from build123d import *
from build123d.topology import SkipClean

# Parameters (mm, degrees)
SKETCH1_R                      = 40
SKETCH1_R_2                    = 38
BOSS_EXTRUDE1_DEPTH            = 200
SKETCH2_R                      = 40
BOSS_EXTRUDE2_DEPTH            = 2
BOSS_EXTRUDE3_DEPTH            = 107
BOSS_EXTRUDE4_DEPTH            = 2
SKETCH5_R                      = 1.75
CUT_EXTRUDE1_DEPTH             = 225.428162226
CUT_EXTRUDE2_REACH             = 218.296
SKETCH6_R                      = 4
CUT_EXTRUDE2_DIRECTION_2_REACH = 218.296
CIRPATTERN1_COUNT              = 2
CIRPATTERN1_ANGLE              = 90
BOSS_EXTRUDE5_REACH            = 241.742
BOSS_EXTRUDE5_END_RADIUS       = 40
SKETCH7_W                      = 14
SKETCH7_H                      = 5
CUT_EXTRUDE3_REACH             = 221.818
SKETCH8_R                      = 1.75
FILLET1_R                      = 3
CUT_EXTRUDE4_REACH             = 220.598
SKETCH9_R                      = 0.25
BOSS_EXTRUDE6_START            = 2
BOSS_EXTRUDE6_DEPTH            = 2
CUT_EXTRUDE5_REACH             = 220.147


with BuildPart() as part:
    # Sketch1 → Boss-Extrude1 (new body)
    with BuildSketch(Plane.XY):
        Circle(SKETCH1_R)
        Circle(SKETCH1_R_2, mode=Mode.SUBTRACT)
    extrude(amount=BOSS_EXTRUDE1_DEPTH)

    # Sketch2 → Boss-Extrude2 (add)
    with BuildSketch(Plane.XY.offset(180)):
        Circle(SKETCH2_R)
    extrude(amount=BOSS_EXTRUDE2_DEPTH)

    # Sketch3 → Boss-Extrude3 (add)
    with BuildSketch(Plane(origin=(0, 0, 0), x_dir=(-1, 0, 0), z_dir=(0, 0, -1))):
        with BuildLine():
            Line((-24, -32), (-72, -32))
            Line((-72, -32), (-72, -30))
            Line((-72, -30), (-26.457513111, -30))
            ThreePointArc((-26.457513111, -30), (-25.248567431, -31.024342744), (-24, -32))
        make_face()
        with BuildLine():
            Line((-24, 32), (-72, 32))
            Line((-72, 32), (-72, 30))
            Line((-72, 30), (-26.457513111, 30))
            ThreePointArc((-26.457513111, 30), (-25.248567431, 31.024342744), (-24, 32))
        make_face()
    extrude(amount=-BOSS_EXTRUDE3_DEPTH)

    # Sketch4 → Boss-Extrude4 (add)
    with BuildSketch(Plane.XY.offset(107)):
        with BuildLine():
            Line((72, -32), (24, -32))
            ThreePointArc((24, -32), (40, 0), (24, 32))
            Line((24, 32), (72, 32))
            Line((72, 32), (72, -32))
        make_face()
    extrude(amount=BOSS_EXTRUDE4_DEPTH)

    # Sketch5 → Cut-Extrude1 (cut, through all)
    with BuildSketch(Plane(origin=(0, 32, 0), x_dir=(1, 0, 0), z_dir=(0, 1, 0))):
        with Locations(Location((43.5, -102.5, 0), (0, 0, 270))):
            Circle(SKETCH5_R)
        with Locations(Location((43.5, -3.5, 0), (0, 0, 270))):
            Circle(SKETCH5_R)
        with Locations(Location((68.5, -78, 0), (0, 0, 270))):
            Circle(SKETCH5_R)
    extrude(amount=-CUT_EXTRUDE1_DEPTH, mode=Mode.SUBTRACT)

    # Sketch6 → Cut-Extrude2 (cut, up to next)
    with BuildSketch(Plane(origin=(0, 0, 0), x_dir=(0, 0, 1), z_dir=(-0.7071067811865488, 0.7071067811865464, 0)), mode=Mode.PRIVATE) as cut_extrude2_sk1:
        with Locations(Location((187, 0, 0), (0, 0, 90))):
            Circle(SKETCH6_R)
    cut_extrude2_tool1 = extrude(cut_extrude2_sk1.sketch, amount=-CUT_EXTRUDE2_REACH, mode=Mode.PRIVATE) & part.part
    cut_extrude2 = cut_extrude2_tool1.solids().sort_by_distance((0, 0, 187))[0]
    add(cut_extrude2, mode=Mode.SUBTRACT)

    # Sketch6 → Cut-Extrude2 direction 2 (cut, up to next)
    with BuildSketch(Plane(origin=(0, 0, 0), x_dir=(0, 0, 1), z_dir=(-0.7071067811865488, 0.7071067811865464, 0)), mode=Mode.PRIVATE) as cut_extrude2_direction_2_sk1:
        with Locations(Location((187, 0, 0), (0, 0, 90))):
            Circle(SKETCH6_R)
    cut_extrude2_direction_2_tool1 = extrude(cut_extrude2_direction_2_sk1.sketch, amount=CUT_EXTRUDE2_DIRECTION_2_REACH, mode=Mode.PRIVATE) & part.part
    cut_extrude2_direction_2 = cut_extrude2_direction_2_tool1.solids().sort_by_distance((0, 0, 187))[0]
    add(cut_extrude2_direction_2, mode=Mode.SUBTRACT)

    # CirPattern1: Cut-Extrude2, Cut-Extrude2 direction 2 ×2 about axis
    cirpattern1_axis = Axis((0, 0, -12.1), (0, 0, 1))
    add([cut_extrude2.rotate(cirpattern1_axis, i * CIRPATTERN1_ANGLE / (CIRPATTERN1_COUNT - 1)) for i in range(1, CIRPATTERN1_COUNT)], mode=Mode.SUBTRACT)
    add([cut_extrude2_direction_2.rotate(cirpattern1_axis, i * CIRPATTERN1_ANGLE / (CIRPATTERN1_COUNT - 1)) for i in range(1, CIRPATTERN1_COUNT)], mode=Mode.SUBTRACT)

    # Boss-Extrude5: up to this cylinder (the profile starts outside it)
    boss_extrude5_end = Plane(origin=(0, 0, 7), z_dir=(0, 0, -1)) * Cylinder(BOSS_EXTRUDE5_END_RADIUS, 564.484, mode=Mode.PRIVATE)
    # Sketch7 → Boss-Extrude5 (add, up to the surface)
    with BuildSketch(Plane(origin=(-54, 0, 0), x_dir=(0, 0, -1), z_dir=(1, 0, 0)), mode=Mode.PRIVATE) as boss_extrude5_sk1:
        with Locations((-7, -13.5)):
            Rectangle(SKETCH7_W, SKETCH7_H)
    boss_extrude5_tool1 = extrude(boss_extrude5_sk1.sketch, amount=BOSS_EXTRUDE5_REACH, mode=Mode.PRIVATE) - boss_extrude5_end
    add(boss_extrude5_tool1.solids().sort_by_distance((-54, -13.5, 7))[0])
    # Sketch7 → Boss-Extrude5 (add, up to the surface)
    with BuildSketch(Plane(origin=(-54, 0, 0), x_dir=(0, 0, -1), z_dir=(1, 0, 0)), mode=Mode.PRIVATE) as boss_extrude5_sk2:
        with Locations((-7, 13.5)):
            Rectangle(SKETCH7_W, SKETCH7_H)
    boss_extrude5_tool2 = extrude(boss_extrude5_sk2.sketch, amount=BOSS_EXTRUDE5_REACH, mode=Mode.PRIVATE) - boss_extrude5_end
    add(boss_extrude5_tool2.solids().sort_by_distance((-54, 13.5, 7))[0])

    # Cut-Extrude3: up to this face of the body (flat: up to its plane)
    cut_extrude3_end = Plane(part.part.faces().sort_by_distance((-45.33030278, 16, 7))[0])
    # Sketch8 → Cut-Extrude3 (cut, up to the picked face)
    with BuildSketch(Plane.XZ.offset(16), mode=Mode.PRIVATE) as cut_extrude3_sk1:
        with Locations(Location((-50, 5, 0), (0, 0, 270))):
            Circle(SKETCH8_R)
    cut_extrude3_tool1 = split(extrude(cut_extrude3_sk1.sketch, amount=-CUT_EXTRUDE3_REACH, mode=Mode.PRIVATE), bisect_by=cut_extrude3_end, keep=Keep.BOTH, mode=Mode.PRIVATE)
    add(cut_extrude3_tool1.solids().sort_by(Axis((-50, -16, 5), (0, 1, 0)))[0], mode=Mode.SUBTRACT)

    # Fillet1
    fillet1_edges = [part.edges().sort_by_distance(p)[0] for p in [
        (-54, -13.5, 14),
        (-54, -13.5, 0),
        (-54, 13.5, 0),
        (-54, 13.5, 14),
    ]]
    fillet(fillet1_edges, radius=FILLET1_R)

    # Sketch9 → Cut-Extrude4 (cut, up to next)
    with BuildSketch(Plane.XZ.offset(-11), mode=Mode.PRIVATE) as cut_extrude4_sk1:
        with Locations(Location((-44, 7, 0), (0, 0, 270))):
            Circle(SKETCH9_R)
    cut_extrude4_tool1 = extrude(cut_extrude4_sk1.sketch, amount=-CUT_EXTRUDE4_REACH, mode=Mode.PRIVATE) & part.part
    add(cut_extrude4_tool1.solids().sort_by_distance((-44, 11, 7))[0], mode=Mode.SUBTRACT)

    # Sketch10 → Boss-Extrude6 (add)
    with SkipClean():  # the faces are left unmerged after this step: merging them gives an invalid solid
        with BuildSketch(Plane(origin=(0, 0, 0), x_dir=(-1, 0, 0), z_dir=(0, 0, -1)).offset(BOSS_EXTRUDE6_START)):
            with BuildLine():
                ThreePointArc((10, -36.66060556), (0, -38), (-10, -36.66060556))
                Line((-10, -36.66060556), (-10, -38.729833462))
                ThreePointArc((-10, -38.729833462), (0, -40), (10, -38.729833462))
                Line((10, -38.729833462), (10, -36.66060556))
            make_face()
            with BuildLine():
                ThreePointArc((10, 38.729833462), (0, 40), (-10, 38.729833462))
                Line((-10, 38.729833462), (-10, 36.66060556))
                ThreePointArc((-10, 36.66060556), (0, 38), (10, 36.66060556))
                Line((10, 36.66060556), (10, 38.729833462))
            make_face()
        extrude(amount=-BOSS_EXTRUDE6_DEPTH)

    # Sketch11 → Cut-Extrude5 (cut, up to next)
    with BuildSketch(Plane.XY.offset(200), mode=Mode.PRIVATE) as cut_extrude5_sk1:
        with BuildLine():
            ThreePointArc((14.062684519, 37.446507235), (-20.975291487, 34.059318065), (-39.768785027, 4.294617267))
            ThreePointArc((-39.768785027, 4.294617267), (-57.533773757, -120.199175418), (66.76517374, -101.118533584))
            ThreePointArc((66.76517374, -101.118533584), (210.736936915, 32.945452835), (14.062684519, 37.446507235))
        make_face()
    cut_extrude5_tool1 = extrude(cut_extrude5_sk1.sketch, amount=-CUT_EXTRUDE5_REACH, mode=Mode.PRIVATE) & part.part
    add(cut_extrude5_tool1.solids().sort_by_distance((72.535197, -23.225739, 200))[0], mode=Mode.SUBTRACT)


solid = part.part
Part model, mm, in its own coordinate system. Coordinates: 2 decimals unless noted, no trailing zeros. Order: outer loops, then holes, each group sorted by start corner. A loop starts at its lowest first (then second) coordinate and runs counter-clockwise, first axis right, second up. Notation, with made-up numbers: M -21,80.25 L 15,80.25 A12 ccw 15,101.25 Z; hole C -1,13 d9. An arc over 180 degrees is marked long. One line per question, with ' | ' between items.
Q1. Two-plate mould, pull along X, no slides. Class faces 1 (the face through (-54, 14, 7)), 2 (the face through (-51.71, 13.46, 5.38)), 3 (the face through (-44, 13, 14)): +X half, -X half, draft (parallel to the pull), parting line (faces both ways), or undercut.
A:
face 1: -X half | face 2: undercut | face 3: draft
Q2. Slice it at A-A (x = -50). Give the cut face in (y, z).
A:
outline: M 11,0 L 16,0 L 16,3.25 L 11,3.25 Z; M 11,6.75 L 16,6.75 L 16,14 L 11,14 Z
Q3. Slice it at C-C (y = 14.55). Give the cut face in (x, z), and give its area (3 significant figures).
A:
outline: M -54,3 A3 ccw -51,0 L -37.26,0 L -37.26,14 L -51,14 A3 ccw -54,11 Z; hole C -50,5 d3.5; hole C -44,7 d0.5 | area: 221 mm^2
Q4. Drill centre lines: line 1 (Z direction, x = -44, y = 13.9); line 2 (X direction, y = 12.4, z = 7); line 3 (X direction, y = 14.7, z = 7). Where is each one in solid material? Low to high.
A:
line 1: z = 0 to 6.75, 7.25 to 14 | line 2: x = -54 to -44.25, -43.75 to -38.03 | line 3: x = -54 to -44.25, -43.75 to -37.2
Q5. Slice it at D-D (y = 12.65). Give the cut face in (x, z), and give its area (3 significant figures).
A:
outline: M -54,3 A3 ccw -51,0 L -37.95,0 L -37.95,14 L -51,14 A3 ccw -54,11 Z; hole C -50,5 d3.5; hole C -44,7 d0.5 | area: 211 mm^2
Q6. Slice it at B-B (z = 7). Give the cut face in (x, y).
A:
outline: M -54,11 L -44.25,11 L -44.25,16 L -54,16 Z; M -43.75,11 L -38.46,11 A40 cw -36.66,16 L -43.75,16 Z
